```python
from build123d import *

# Parameters (mm, degrees)
F0_W     = 1016
F0_H     = 838.2
F1_DEPTH = 19.05
F2_W     = 12.7
F2_H     = 152.4
F2_W_2   = 19.05
F2_W_3   = 203.2
F2_H_2   = 19.05
F3_DEPTH = 19.051
F4_W     = 203.2
F4_H     = 6.35
F4_W_2   = 6.35
F4_H_2   = 152.4
F5_DEPTH = 19.05
F6_W     = 6.35
F6_H     = 152.4
F7_DEPTH = 19.051


with BuildPart() as f1:
    # F0 (on Top) → F1 (new body)
    with BuildSketch(Plane.XY):
        with Locations((-104.35828, 419.1)):
            Rectangle(F0_W, F0_H)
    extrude(amount=F1_DEPTH)

    # F2 (on face) → F3 (cut, through all)
    with BuildSketch(Plane.XY.offset(19.05)):
        with Locations((397.29172, 266.7)):
            Rectangle(F2_W, F2_H)
        with Locations((394.11672, 571.5)):
            Rectangle(F2_W_2, F2_H)
        with Locations((-606.00828, 266.7)):
            Rectangle(F2_W, F2_H)
        with Locations((-606.00828, 571.5)):
            Rectangle(F2_W, F2_H)
        with Locations((-307.55828, 9.525)):
            Rectangle(F2_W_3, F2_H_2)
        with Locations((98.84172, 9.525)):
            Rectangle(F2_W_3, F2_H_2)
        with Locations((98.84172, 828.675)):
            Rectangle(F2_W_3, F2_H_2)
        with Locations((-307.55828, 828.675)):
            Rectangle(F2_W_3, F2_H_2)
    extrude(amount=-F3_DEPTH, mode=Mode.SUBTRACT)

    # F4 (on face) → F5 (join)
    with BuildSketch(Plane.XY.offset(19.05)):
        with Locations((-510.75828, 841.375)):
            Rectangle(F4_W, F4_H)
        with Locations((98.84172, 822.325)):
            Rectangle(F4_W, F4_H)
        with Locations((-307.55828, 822.325)):
            Rectangle(F4_W, F4_H)
        with Locations((-104.35828, 841.375)):
            Rectangle(F4_W, F4_H)
        with Locations((302.04172, 841.375)):
            Rectangle(F4_W, F4_H)
        with Locations((-307.55828, 15.875)):
            Rectangle(F4_W, F4_H)
        with Locations((-510.75828, -3.175)):
            Rectangle(F4_W, F4_H)
        with Locations((98.84172, 15.875)):
            Rectangle(F4_W, F4_H)
        with Locations((302.04172, -3.175)):
            Rectangle(F4_W, F4_H)
        with Locations((-104.35828, -3.175)):
            Rectangle(F4_W, F4_H)
        with Locations((-596.48328, 266.7)):
            Rectangle(F4_W_2, F4_H_2)
        with Locations((-596.48328, 571.5)):
            Rectangle(F4_W_2, F4_H_2)
        with Locations((387.76672, 266.7)):
            Rectangle(F4_W_2, F4_H_2)
        with Locations((381.41672, 571.5)):
            Rectangle(F4_W_2, F4_H_2)
    extrude(amount=-F5_DEPTH)

    # F6 (on face) → F7 (cut, through all)
    with BuildSketch(Plane.XY.offset(19.05)):
        with Locations((-596.48328, 571.5)):
            Rectangle(F6_W, F6_H)
        with Locations((-596.48328, 266.7)):
            Rectangle(F6_W, F6_H)
        with Locations((387.76672, 266.7)):
            Rectangle(F6_W, F6_H)
        with Locations((387.76672, 571.5)):
            Rectangle(F6_W, F6_H)
    extrude(amount=-F7_DEPTH, mode=Mode.SUBTRACT)


solid = f1.part
```
Work out the finished part from the listing and answer in its coordinate system (mm). Coordinates: 2 decimals unless noted, no trailing zeros. Write each loop counter-clockwise with the first axis right and the second up, starting at its lowest first coordinate (ties: lowest second). Pieces come first, ordered by that corner, then holes.
Q1. Each of these flat-tipped pins is pushed along its axis until it touches: pin 1 Ø5 at (x, z) = (-331, 6) entering from -Y; pin 2 Ø9.5 at (y, z) = (245, 13.5) entering from -X; pin 3 Ø5.5 at (y, z) = (551, 5) entering from +X. Where does it stop, or does it pass through?
Q2. Find the intervals of material crossed by line 1 (Y direction, x = -260, z = 3); line 2 (X direction, y = 331, z = 11.5), in increasing order.
Q3. A cutting plane is placed at A-A, the plane x = -255. Give the vertices of the cut face in (y, z).
Findings below:
1. pin 1: stops at y = 12.7
1. pin 2: stops at x = -593.31
1. pin 3: stops at x = 384.59
2. line 1: y = 12.7 to 825.5
2. line 2: x = -593.31 to 384.59
3. outline: (12.7, 0) - (825.5, 0) - (825.5, 19.05) - (12.7, 19.05) - close
